from build123d import *

# Parameters (mm, degrees)
F1_DEPTH = 50.8
F3_DEPTH = 12.7
F4_W     = 12.7
F4_H     = 19.05
F5_DEPTH = 19.05
F7_DEPTH = 12.7


with BuildPart() as f1:
    # F0 (on Right) → F1 (new body)
    with BuildSketch(Plane.YZ):
        Polygon((0, 12.7), (0, 0), (31.75, 0), (31.75, 31.75), (19.05, 31.75), (19.05, 12.7), align=None)
    extrude(amount=F1_DEPTH)

    # F2 (on face) → F3 (cut)
    with BuildSketch(Plane.XZ.offset(-19.05)):
        Polygon((50.8, 31.75), (33.761162, 31.75), (50.8, 12.7), align=None)
    extrude(amount=-F3_DEPTH, mode=Mode.SUBTRACT)

    # F4 (on face) → F5 (join)
    with BuildSketch(Plane.XZ.offset(-19.05)):
        with Locations((25.4, 22.225)):
            Rectangle(F4_W, F4_H)
    extrude(amount=F5_DEPTH)

    # F6 (on face) → F7 (cut)
    with BuildSketch(Plane.YZ.offset(31.75)):
        Polygon((0, 12.7), (19.05, 31.75), (0, 31.75), align=None)
    extrude(amount=-F7_DEPTH, mode=Mode.SUBTRACT)


solid = f1.part
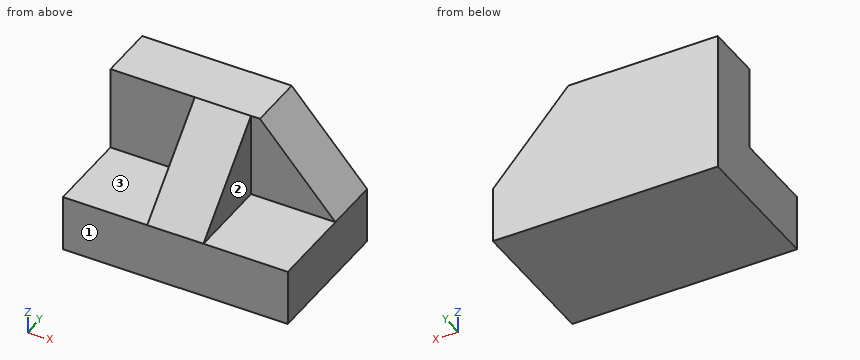
CAD build for the part. Positions are in the model's coordinates, mm. Face numbers are marked on the shaded views. A direction names the side the tool comes from. Round coordinates to 2 decimals unless told otherwise and drop trailing zeros. Write each loop counter-clockwise with the first axis right and the second up, starting at its lowest first coordinate (ties: lowest second). Pieces come first, ordered by that corner, then holes. Notation, with made-up numbers: M 43.25,60.5 L 60.25,60.5 A18 ccw 60.25,91.5 Z; hole C -8,10.5 d8. An arc over 180 degrees is marked long. Use a Markdown table: item, result. Add a question column.
1. Drill centre lines: probe 1 along Y at (x, z) = (13, 23); probe 2 along Z at (x, y) = (15.5, 15). Where is each one in solid material? Low to high.
2. Slice it at D-D on x = 5.5. Give the cut face in (y, z).
3. Flat gauge pins, fed straight in: P1, Ø10, axis at y = 9.5, z = 3.5, coming from the -X side; P2, Ø9.5, axis at x = 41, y = 6.5, coming from the +Z side; P3, Ø9.5, axis at x = 9, z = 20, coming from the -Y side; P4, Ø9.5, axis at y = 10, z = 23, coming from the -X side. Where does each tip first touch, or does it go through?
4. Slice it at C-C on z = 14. Give the cut face in (x, y), then the cut area to 3 significant figures.
5. Slice it at B-B on y = 14. Give the cut face in (x, z), then the cut area to 3 significant figures.
6. 3-axis set-ups, long thin cutter, end or side, ignore diameter. For the marked faces 1, 2 and 3: which of +Z, -Z, +X, -X, +Y, -Y reach the whole face in a straight line?
7. Slice it at A-A on x = 23. Give the cut face in (y, z).
Reply:
| question | item | result |
|---|---|---|
| 1 | probe 1 | y = 19.05 to 31.75 |
| 1 | probe 2 | z = 0 to 12.7 |
| 2 | outline | M 0,0 L 31.75,0 L 31.75,31.75 L 19.05,31.75 L 19.05,12.7 L 0,12.7 Z |
| 3 | P1 | stops at x = 0 |
| 3 | P2 | stops at z = 12.7 |
| 3 | P3 | stops at y = 19.05 |
| 3 | P4 | stops at x = 19.05 |
| 4 | outline | M 0,19.05 L 19.05,19.05 L 19.05,1.3 L 31.75,1.3 L 31.75,19.05 L 49.64,19.05 L 49.64,31.75 L 0,31.75 Z |
| 4 | area | 856 mm^2 |
| 5 | outline | M 0,0 L 50.8,0 L 50.8,12.7 L 31.75,12.7 L 31.75,26.7 L 19.05,26.7 L 19.05,12.7 L 0,12.7 Z |
| 5 | area | 823 mm^2 |
| 6 | face 1 | +Z, -Z, +X, -X, -Y |
| 6 | face 2 | +Z, +X, -Y |
| 6 | face 3 | +Z, -X, -Y |
| 7 | outline | M 0,0 L 31.75,0 L 31.75,31.75 L 19.05,31.75 L 0,12.7 Z |
